from build123d import *
from build123d.topology import SkipClean

# Parameters (mm, degrees)
REVOLVE1_ANGLE               = 180
BOSS_EXTRUDE1_DEPTH          = 22
BOSS_EXTRUDE1_DEPTH_BACK     = 5
SKETCH3_R                    = 0.875
BOSS_EXTRUDE2_DEPTH          = 5
BOSS_EXTRUDE2_DEPTH_BACK     = 5
SKETCH4_W                    = 4.7
SKETCH4_H                    = 9.1
CUT_REVOLVE1_ANGLE           = 9
CUT_REVOLVE1_OTHER_WAY_ANGLE = 9


with BuildPart() as part:
    # Sketch1 → Revolve1 (revolve)
    with BuildSketch(Plane.XY):
        with BuildLine():
            Line((0, 27.259159134), (23.011868121, 27.259159134))
            ThreePointArc((23.011868121, 27.259159134), (27.855738892, 24.833992365), (28.816239605, 19.502767713))
            ThreePointArc((28.816239605, 19.502767713), (27.949144344, 9.543519717), (31.011361688, 0.027149624))
            ThreePointArc((31.011361688, 0.027149624), (32.915416284, -3.265823742), (34.05, -6.89650099))
            Line((34.05, -6.89650099), (34.05, -36.726991211))
            Line((34.05, -36.726991211), (0, -36.726991211))
            Line((0, -36.726991211), (0, -38.526991211))
            Line((0, -38.526991211), (35.85, -38.526991211))
            Line((35.85, -38.526991211), (35.85, 29.059159134))
            Line((35.85, 29.059159134), (0, 29.059159134))
            Line((0, 29.059159134), (0, 27.259159134))
        make_face()
    revolve(axis=Axis((0, 0, 0), (0, 1, 0)), revolution_arc=REVOLVE1_ANGLE)

    # Sketch3 → Boss-Extrude1 (add, two sides: drawn at the far end of the back side and taken through both)
    with BuildSketch(Plane(origin=(0, 0, 0), x_dir=(1, 0, 0), z_dir=(0, 1, 0)).offset(-BOSS_EXTRUDE1_DEPTH_BACK)):
        with BuildLine():
            Line((-35.835435362, 1.02179861), (-35.66522342, 1.724252792))
            Line((-35.66522342, 1.724252792), (-35.552792373, 4.606674994))
            ThreePointArc((-35.552792373, 4.606674994), (-36.966498022, 3.313002301), (-38.45, 2.1))
            ThreePointArc((-38.45, 2.1), (-39.934924016, -1.484924465), (-36.35, 6.34e-07))
            ThreePointArc((-36.35, 6.34e-07), (-36.156829024, 0.54318529), (-35.835435362, 1.02179861))
        make_face()
        with Locations(Location((-38.45, 0, 0), (0, 0, 270))):
            Circle(SKETCH3_R, mode=Mode.SUBTRACT)
    extrude(amount=BOSS_EXTRUDE1_DEPTH + BOSS_EXTRUDE1_DEPTH_BACK)

    # Sketch5 → Boss-Extrude2 (add, two sides: drawn at the far end of the back side and taken through both)
    with BuildSketch(Plane(origin=(0, 0, 0), x_dir=(1, 0, 0), z_dir=(0, 1, 0)).offset(-BOSS_EXTRUDE2_DEPTH_BACK)):
        with BuildLine():
            Line((36.194622224, -1.309022975), (35.85, 0))
            ThreePointArc((35.85, 0), (35.761021608, 2.524249113), (35.494528112, 5.035968037))
            Line((35.494528112, 5.035968037), (38.337267345, 3.105755306))
            ThreePointArc((38.337267345, 3.105755306), (38.578712242, 2.836355157), (38.665960295, 2.485271326))
            Line((38.665960295, 2.485271326), (38.665960295, -2.467611774))
            ThreePointArc((38.665960295, -2.467611774), (38.519513686, -2.821165165), (38.165960295, -2.967611774))
            Line((38.165960295, -2.967611774), (37.169410283, -2.967611774))
            Line((37.169410283, -2.967611774), (36.551786147, -2.967611774))
            ThreePointArc((36.551786147, -2.967611774), (36.48188919, -2.945153638), (36.438154821, -2.886185362))
            Line((36.438154821, -2.886185362), (36.415143378, -2.818397505))
            ThreePointArc((36.415143378, -2.818397505), (36.933237669, -1.971906955), (36.194622224, -1.309022975))
        make_face()
    extrude(amount=BOSS_EXTRUDE2_DEPTH + BOSS_EXTRUDE2_DEPTH_BACK)

    # Sketch4 → Cut-Revolve1 (revolve, cut)
    with BuildSketch(Plane.XY):
        with Locations((-38.2, 8.5)):
            Rectangle(SKETCH4_W, SKETCH4_H)
    revolve(axis=Axis((0, 0, 0), (0, 1, 0)), revolution_arc=CUT_REVOLVE1_ANGLE, mode=Mode.SUBTRACT)

    # Sketch4 → Cut-Revolve1 other way (revolve, cut)
    with SkipClean():  # the faces are left unmerged after this step: merging them gives an invalid solid
        with BuildSketch(Plane.XY):
            with Locations((-38.2, 8.5)):
                Rectangle(SKETCH4_W, SKETCH4_H)
        revolve(axis=Axis((0, 0, 0), (0, -1, 0)), revolution_arc=CUT_REVOLVE1_OTHER_WAY_ANGLE, mode=Mode.SUBTRACT)


solid = part.part
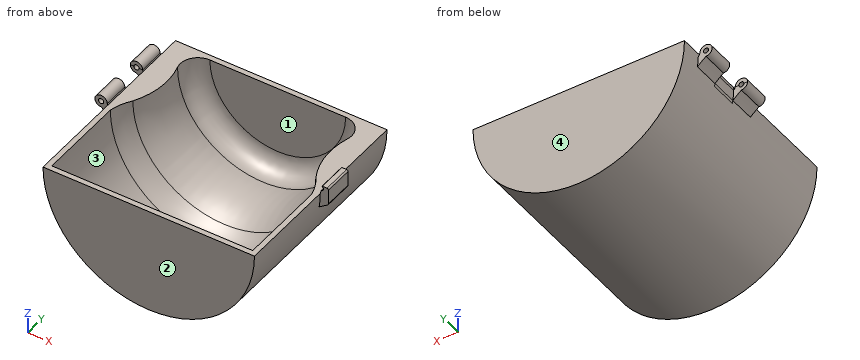
Verification items for the finished model (mm, model axes). Face numbers are marked on the shaded views. A direction names the side the tool comes from. Round coordinates to 2 decimals unless told otherwise and drop trailing zeros. Loops run counter-clockwise (first coordinate to the right, second up) from the corner with the lowest first, then second, coordinate; pieces in that order, holes last. Notation, with made-up numbers: (11, 19) - (57, 19) arc R14 ccw to (57, 27) - close; hole circle Ø11 at (79, 55.25). An arc over 180 degrees is marked (long way). Answer in a Markdown table with one row per item. Add a question column.
Q1. Release check for a two-part mould opening along X. For the marked faces 1 and 2 record: pulls with the +X half, pulls with the -X half, needs draft (parallel to the pull), parting line crosses it, or undercut.
Q2. Material ranges on line 1 (Z direction, x = -38.45, y = 17.75) (3 decimals); line 2 (Y direction, x = 7, z = -7); line 3 (Y direction, x = -14, z = -30), recorded low to high.
Q3. Gauge pin test, flat ends, axial feed: pin 1 (2 mm diameter, centred on y = -27.5, z = -10, fed in from +X); pin 2 (2 mm diameter, centred on y = -28, z = -22, fed in from +X); pin 3 (2.5 mm diameter, centred on x = -38.5, z = 1, fed in from +Y). Record the tip position at first contact, or that the pin passes through.
Q4. Section check A-A on y = -21.5. Enter the section's corners in (x, z), plus the area to 3 significant figures.
Q5. Section check B-B on z = -28. State how many separate pieces and enclosed holes the cut face has, plus the area to 3 significant figures.
Q6. Tool access check on the marked faces 3 and 4. Record the directions out of +Z, -Z, +X, -X, +Y, -Y that give a thin tool (end or side, any length) a straight path to the whole face; none if there is none.
Found:
| question | item | result |
|---|---|---|
| 1 | face 1 | undercut |
| 1 | face 2 | needs draft |
| 2 | line 1 | z = -2.1 to -0.875, 0.875 to 2.1 |
| 2 | line 2 | y = -38.53 to -36.73, 27.26 to 29.06 |
| 2 | line 3 | y = -38.53 to -36.73, -3.72 to 29.06 |
| 3 | pin 1 | stops at x = 34.7 |
| 3 | pin 2 | stops at x = 29.06 |
| 3 | pin 3 | stops at y = 22 |
| 4 | outline | (-35.85, 0) arc R35.85 ccw to (35.85, 0) - (34.05, 0) arc R34.05 cw to (-34.05, 0) - close |
| 4 | area | 198 mm² |
| 5 | separate pieces | 1 |
| 5 | enclosed holes | 2 |
| 5 | area | 1,400 mm² |
| 6 | face 3 | +Z |
| 6 | face 4 | +Z, -Z, +X, -X, +Y |
